For this review, take the finished solid that the model builds, in its own axes (mm). A direction names the side the tool comes from. Coordinates: 2 decimals unless noted, no trailing zeros. Order: outer loops, then holes, each group sorted by start corner. A loop starts at its lowest first (then second) coordinate and runs counter-clockwise, first axis right, second up. Notation, with made-up numbers: (-24.5, 86.5) - (3.5, 86.5) arc R19 ccw to (3.5, 116.5) - close; hole circle Ø6 at (24.5, 62). An arc over 180 degrees is marked (long way). One line per item, written item: value. Start each with the question number.
(1) Consider section C-C on x = -8.5. Write out the cut boundary in (y, z), then the cut area to 3 significant figures.
(2) Consider section D-D on x = -16. Write out the cut boundary in (y, z).
(3) Consider section A-A on y = 13. Write out the cut boundary in (x, z) (3 decimals).
(4) Clearance check with flat-ended pins moving along their axes: pin 1 (1.8 mm diameter, centred on x = 4.375, z = 15, fed in from +Y); pin 2 (1 mm diameter, centred on x = -47.5, z = 12, fed in from +Y); pin 3 (11.5 mm diameter, centred on y = 4, z = 13, fed in from -X); pin 4 (2.5 mm diameter, centred on y = -25, z = 22.5, fed in from -X). State where each tip first meets the part, or that it passes through.
(5) To check wall thickness, follow line 1 along Z through (x, y) = (-8.5, 11); line 2 along Y through (x, z) = (0, 13.5); line 3 along X through (y, z) = (17.5, 15) (3 decimals). State the ranges of each line that lie inside material, in increasing order.
(6) For faces 4 (the cylindrical face through (5.715, -8.681, 14.944)), 5 (the flat face through (6.3, -22.5, 19.9)), 6 (the flat face through (-2.5, 11, 23)), 7 (the flat face through (-50, -13.85, 2)), list the 3-axis set-ups (+Z, -Z, +X, -X, +Y, -Y) from which the entire face can be reached by the end or side of a thin tool; tool diameter is ignored.
(7) Mouldability with a two-part tool opening along X and no side actions: class faces 1 (the flat face through (-11, -25, 17)), 2 (the flat face through (-45.5, -16, 2)), 3 (the flat face through (-5.951, 16.146, 10.351)) as released by +X, released by -X, zero draft, split by the parting line, or undercut.
(8) Consider section B-B on y = 0. Write out the cut boundary in (x, z).
```python
from build123d import *

# Parameters (mm, degrees)
SKETCH1_R               = 5
SKETCH1_W               = 9
SKETCH1_H               = 3.3
BOSS_EXTRUDE1_DEPTH     = 28
SKETCH2_W               = 50.5
SKETCH2_H               = 47
CUT_EXTRUDE1_DEPTH      = 23
SKETCH3_R               = 6.65
CUT_EXTRUDE2_DEPTH      = 5
CUT_EXTRUDE3_START      = -5
SKETCH4_R               = 6.65
CUT_EXTRUDE3_DEPTH      = 5
SKETCH5_R               = 12
CUT_EXTRUDE4_DEPTH      = 8
CUT_EXTRUDE5_START      = -9
CUT_EXTRUDE5_DEPTH      = 9
CUT_EXTRUDE6_DEPTH      = 6
SKETCH8_R               = 1.15
CUT_EXTRUDE7_DEPTH      = 85.190260719
CHAMFER1_SIZE           = 21
CHAMFER1_SIZE2          = 50.5
SKETCH9_R               = 2.2
CUT_EXTRUDE8_DEPTH      = 83.137080542
CUT_EXTRUDE9_DEPTH      = 3
CUT_EXTRUDE9_DEPTH_BACK = 7
BOSS_EXTRUDE2_DEPTH     = 10
LPATTERN1_COUNT         = 2
LPATTERN1_PITCH         = 60.5
SKETCH12_R              = 1.75
CUT_EXTRUDE10_DEPTH     = 10
CHAMFER2_SIZE           = 3
CHAMFER3_SIZE           = 1.8


with BuildPart() as part:
    # Sketch1 → Boss-Extrude1 (new body)
    with BuildSketch(Plane.XY):
        with BuildLine():
            Line((-60, -31.5), (10.5, -31.5))
            Line((10.5, -31.5), (10.5, 20.5))
            Line((10.5, 20.5), (-28.5, 20.5))
            Line((-28.5, 20.5), (-28.5, 12.180409823))
            ThreePointArc((-28.5, 12.180409823), (-20.217668105, -2.285689125), (-33, -12.985083113))
            Line((-33, -12.985083113), (-36, -12.985083113))
            ThreePointArc((-36, -12.985083113), (-41.689100041, -11.672468641), (-46.228019527, -8))
            Line((-46.228019527, -8), (-60, -8))
            Line((-60, -8), (-60, -31.5))
        make_face()
        Circle(SKETCH1_R, mode=Mode.SUBTRACT)
        with Locations((-19, 15.5)):
            Rectangle(SKETCH1_W, SKETCH1_H, mode=Mode.SUBTRACT)
        with Locations((-19, -15.5)):
            Rectangle(SKETCH1_W, SKETCH1_H, mode=Mode.SUBTRACT)
        with Locations((-50, -15.5)):
            Rectangle(SKETCH1_W, SKETCH1_H, mode=Mode.SUBTRACT)
    extrude(amount=BOSS_EXTRUDE1_DEPTH)

    # Sketch2 → Cut-Extrude1 (cut)
    with BuildSketch(Plane.XY.offset(28)):
        with Locations((-34.75, -3)):
            Rectangle(SKETCH2_W, SKETCH2_H)
    extrude(amount=-CUT_EXTRUDE1_DEPTH, mode=Mode.SUBTRACT)

    # Sketch3 → Cut-Extrude2 (cut)
    with BuildSketch(Plane.XY.offset(28)):
        Circle(SKETCH3_R)
    extrude(amount=-CUT_EXTRUDE2_DEPTH, mode=Mode.SUBTRACT)

    # Sketch4 → Cut-Extrude3 (cut)
    with BuildSketch(Plane(origin=(0, 0, 0), x_dir=(-1, 0, 0), z_dir=(0, 0, -1)).offset(CUT_EXTRUDE3_START)):
        with Locations(Location((0, 0, 0), (0, 0, 180))):
            Circle(SKETCH4_R)
    extrude(amount=CUT_EXTRUDE3_DEPTH, mode=Mode.SUBTRACT)

    # Sketch5 → Cut-Extrude4 (cut)
    with BuildSketch(Plane.XY.offset(11)):
        with Locations((14, 0)):
            Circle(SKETCH5_R)
    extrude(amount=CUT_EXTRUDE4_DEPTH, mode=Mode.SUBTRACT)

    # Sketch6 → Cut-Extrude5 (cut)
    with BuildSketch(Plane.XZ.offset(31.5).offset(CUT_EXTRUDE5_START)):
        with BuildLine():
            Line((2.725, 15), (2.725, 28))
            Line((2.725, 28), (6.025, 28))
            Line((6.025, 28), (6.025, 15))
            ThreePointArc((6.025, 15), (4.375, 13.35), (2.725, 15))
        make_face()
    extrude(amount=CUT_EXTRUDE5_DEPTH, mode=Mode.SUBTRACT)

    # Sketch7 → Cut-Extrude6 (cut)
    with BuildSketch(Plane.XZ.offset(22.5)):
        Polygon((1.475, 28), (7.275, 28), (7.275, 13.325684219), (4.375, 11.651368439), (1.475, 13.325684219), align=None)
    extrude(amount=-CUT_EXTRUDE6_DEPTH, mode=Mode.SUBTRACT)

    # Sketch8 → Cut-Extrude7 (cut, through all)
    with BuildSketch(Plane.XZ.offset(31.5)):
        with Locations(Location((4.375, 15, 0), (0, 0, 270))):
            Circle(SKETCH8_R)
    extrude(amount=-CUT_EXTRUDE7_DEPTH, mode=Mode.SUBTRACT)

    # Chamfer1
    chamfer1_edges = [part.edges().sort_by_distance(p)[0] for p in [
        (-60, -29, 28),
    ]]
    chamfer1_side = [part.faces().sort_by_distance(p)[0] for p in [
        (-60, -19.75, 0.365547535),
    ]]
    chamfer(chamfer1_edges, length=CHAMFER1_SIZE, length2=CHAMFER1_SIZE2, reference=chamfer1_side[0])

    # Sketch9 → Cut-Extrude8 (cut, through all)
    with BuildSketch(Plane(origin=(10.5, 0, 0), x_dir=(0, 0, -1), z_dir=(1, 0, 0))):
        with Locations((-8.5, 13)):
            Circle(SKETCH9_R)
        with Locations(Location((-21.5, 13, 0), (0, 0, 90))):
            Circle(SKETCH9_R)
        with Locations(Location((-8.5, -13, 0), (0, 0, 90))):
            Circle(SKETCH9_R)
        with Locations((-21.5, -13)):
            Circle(SKETCH9_R)
    extrude(amount=-CUT_EXTRUDE8_DEPTH, mode=Mode.SUBTRACT)

    # Sketch10 → Cut-Extrude9 (cut, two sides: drawn at the far end of the back side and taken through both)
    with BuildSketch(Plane.ZY.offset(9.5).offset(-CUT_EXTRUDE9_DEPTH_BACK)):
        Polygon((4.85, 15.107328483), (4.85, 10.892671517), (8.5, 8.785343035), (12.15, 10.892671517), (12.15, 15.107328483), (8.5, 17.214656965), align=None)
        Polygon((25.15, 10.892671517), (25.15, 15.107328483), (21.5, 17.214656965), (17.85, 15.107328483), (17.85, 10.892671517), (21.5, 8.785343035), align=None)
        Polygon((25.15, -10.892671517), (21.5, -8.785343035), (17.85, -10.892671517), (17.85, -15.107328483), (21.5, -17.214656965), (25.15, -15.107328483), align=None)
        Polygon((12.15, -10.892671517), (8.5, -8.785343035), (4.85, -10.892671517), (4.85, -15.107328483), (8.5, -17.214656965), (12.15, -15.107328483), align=None)
    extrude(amount=CUT_EXTRUDE9_DEPTH + CUT_EXTRUDE9_DEPTH_BACK, mode=Mode.SUBTRACT)

    # Sketch11 → Boss-Extrude2 (add)
    with BuildSketch(Plane(origin=(10.5, 0, 0), x_dir=(0, 0, -1), z_dir=(1, 0, 0))):
        with BuildLine():
            Line((0, -31.5), (-7, -31.5))
            Line((-7, -31.5), (-7, -33.3))
            Line((-7, -33.3), (-5, -33.3))
            ThreePointArc((-5, -33.3), (-1.8, -36.5), (-5, -39.7))
            Line((-5, -39.7), (-7, -39.7))
            Line((-7, -39.7), (-7, -41.5))
            Line((-7, -41.5), (0, -41.5))
            Line((0, -41.5), (0, -31.5))
        make_face()
    boss_extrude2 = extrude(amount=-BOSS_EXTRUDE2_DEPTH)

    # LPattern1: Boss-Extrude2 ×2
    with Locations(*[(-i * LPATTERN1_PITCH, 0, 0) for i in range(1, LPATTERN1_COUNT)]):
        add(boss_extrude2)

    # Sketch12 → Cut-Extrude10 (cut)
    with BuildSketch(Plane(origin=(0, 20.5, 0), x_dir=(1, 0, 0), z_dir=(0, 1, 0))):
        with Locations(Location((4.375, -15, 0), (0, 0, 270))):
            Circle(SKETCH12_R)
    extrude(amount=-CUT_EXTRUDE10_DEPTH, mode=Mode.SUBTRACT)

    # Chamfer2
    chamfer2_edges = [part.edges().sort_by_distance(p)[0] for p in [
        (-9.5, -26.5, 16.5),
    ]]
    chamfer(chamfer2_edges, length=CHAMFER2_SIZE)

    # Chamfer3
    chamfer3_edges = [part.edges().sort_by_distance(p)[0] for p in [
        (-55, -31.5, 7),
        (5.5, -31.5, 7),
    ]]
    chamfer(chamfer3_edges, length=CHAMFER3_SIZE - 0.0001)  # a hair under: the kernel refuses the full size


solid = part.part
```
Geometry check:
1. outline: (-31.5, 0) - (20.5, 0) - (20.5, 28) - (-31.5, 28) - close; hole (-17.21, 8.5) - (-15.11, 4.85) - (-10.89, 4.85) - (-8.79, 8.5) - (-10.89, 12.15) - (-15.11, 12.15) - close; hole (-17.21, 21.5) - (-15.11, 17.85) - (-10.89, 17.85) - (-8.79, 21.5) - (-10.89, 25.15) - (-15.11, 25.15) - close; hole (8.79, 8.5) - (10.89, 4.85) - (15.11, 4.85) - (17.21, 8.5) - (15.11, 12.15) - (10.89, 12.15) - close; hole (8.79, 21.5) - (10.89, 17.85) - (15.11, 17.85) - (17.21, 21.5) - (15.11, 25.15) - (10.89, 25.15) - close
1. area: 1,270 mm^2
2. outline: (-31.5, 0) - (-17.15, 0) - (-17.15, 5) - (-26.5, 5) - (-26.5, 25.3) - (-31.5, 25.3) - close; (-13.85, 0) - (13.85, 0) - (13.85, 5) - (-13.85, 5) - close; (17.15, 0) - (20.5, 0) - (20.5, 5) - (17.15, 5) - close
3. outline: (-28.5, 0) - (10.5, 0) - (10.5, 6.3) - (-2.5, 6.3) - (-2.5, 4.85) - (-12.5, 4.85) - (-12.5, 5) - (-28.5, 5) - close; (-9.5, 12.15) - (-2.5, 12.15) - (-2.5, 10.7) - (10.5, 10.7) - (10.5, 19.3) - (-2.5, 19.3) - (-2.5, 17.85) - (-9.5, 17.85) - close; (-9.5, 25.15) - (-2.5, 25.15) - (-2.5, 23.7) - (10.5, 23.7) - (10.5, 28) - (-9.5, 28) - close; hole circle Ø3.5 at (4.375, 15)
4. pin 1: passes through
4. pin 2: stops at y = -26.5
4. pin 3: stops at x = -9.5
4. pin 4: stops at x = -12.25
5. line 1: z = 0 to 4.85, 12.15 to 17.85, 25.15 to 28
5. line 2: y = -31.5 to -5, 5 to 20.5
5. line 3: x = -9.5 to 2.625, 6.125 to 10.5
6. face 4: +X
6. face 5: +Z
6. face 6: -X
6. face 7: +Z, -Z
7. face 1: released by -X
7. face 2: undercut
7. face 3: zero draft
8. outline: (-20.01, 0) - (-6.65, 0) - (-6.65, 5) - (-5, 5) - (-5, 23) - (-6.65, 23) - (-6.65, 28) - (-9.5, 28) - (-9.5, 5) - (-20.01, 5) - close; (5, 5) - (6.65, 5) - (6.65, 0) - (10.5, 0) - (10.5, 11) - (5, 11) - close; (5, 19) - (10.5, 19) - (10.5, 28) - (6.65, 28) - (6.65, 23) - (5, 23) - close
